Input: part model. Units: mm. Frame: model coordinates. Face numbers are marked on the shaded views. A direction names the side the tool comes from. Coordinates: 2 decimals unless noted, no trailing zeros. Write each loop counter-clockwise with the first axis right and the second up, starting at its lowest first coordinate (ties: lowest second). Pieces come first, ordered by that corner, then holes. Notation, with made-up numbers: (12, -1) - (70, -1) arc R16 cw to (70, 29) - close; hole circle Ø8 at (34.25, -13.75). An arc over 180 degrees is marked (long way). One line per question, with ' | ' between items. Start each with the question number.
1) First-contact query: P1, Ø5.5, axis at x = 0, y = 12, coming from the -Z side; P2, Ø1.2, axis at x = -24, y = 24, coming from the -Z side. Flat tips, straight axial feed; report the tip coordinate or a pass-through.
2) Section query D-D on x = -26.5. Return loops of the section in (y, z).
3) Draft query along Y for the marked faces 1, 2 and 3. Return one class per face: released by +Y, released by -Y, zero draft, split by the parting line, or undercut.
4) Section query A-A on y = 24. Return loops of the section in (x, z) (3 decimals), and give its area (3 significant figures).
5) Section query C-C on z = 4. Give the number of separate pieces and of enclosed holes in the cut face, and give its area (3 significant figures).
6) Reachability of the marked faces 4 and 5 from +Z, -Z, +X, -X, +Y, -Y: full face, straight path, thin tool, end or side. Return the list, or none.
7) Line query: line 1 (Y direction, x = -24, z = 4.75) (3 decimals); line 2 (Y direction, x = -24, z = 0.8); line 3 (X direction, y = 3, z = 1.5). Output: solid intervals per line, ascending.
8) Section query B-B on x = -12. Return loops of the section in (y, z) (3 decimals), and give its area (3 significant figures).
```python
from build123d import *

# Parameters (mm, degrees)
SKETCH1_W           = 40
SKETCH1_H           = 40
SKETCH1_R           = 4.55
BOSS_EXTRUDE1_DEPTH = 1.6
SKETCH2_W           = 40
SKETCH2_H           = 40
SKETCH2_R           = 1.025
BOSS_EXTRUDE2_DEPTH = 15


with BuildPart() as part:
    # Sketch1 → Boss-Extrude1 (new body)
    with BuildSketch(Plane(origin=(0, 0, 0), x_dir=(0, 1, 0), z_dir=(0, 0, 1))):
        with Locations((12, 12)):
            Rectangle(SKETCH1_W, SKETCH1_H)
        with Locations(Location((0, 0, 0), (0, 0, 270))):
            Circle(SKETCH1_R, mode=Mode.SUBTRACT)
        with Locations(Location((12, 0, 0), (0, 0, 270))):
            Circle(SKETCH1_R, mode=Mode.SUBTRACT)
        with Locations(Location((24, 0, 0), (0, 0, 270))):
            Circle(SKETCH1_R, mode=Mode.SUBTRACT)
        with Locations(Location((12, 12, 0), (0, 0, 270))):
            Circle(SKETCH1_R, mode=Mode.SUBTRACT)
        with Locations(Location((24, 12, 0), (0, 0, 270))):
            Circle(SKETCH1_R, mode=Mode.SUBTRACT)
        with Locations(Location((12, 24, 0), (0, 0, 270))):
            Circle(SKETCH1_R, mode=Mode.SUBTRACT)
        with Locations(Location((24, 24, 0), (0, 0, 270))):
            Circle(SKETCH1_R, mode=Mode.SUBTRACT)
        with Locations(Location((0, 12, 0), (0, 0, 270))):
            Circle(SKETCH1_R, mode=Mode.SUBTRACT)
        with Locations(Location((0, 24, 0), (0, 0, 270))):
            Circle(SKETCH1_R, mode=Mode.SUBTRACT)
    extrude(amount=BOSS_EXTRUDE1_DEPTH)

    # Sketch2 → Boss-Extrude2 (add)
    with BuildSketch(Plane.XY.offset(1.6)):
        with Locations((-12, 12)):
            Rectangle(SKETCH2_W, SKETCH2_H)
        Circle(SKETCH2_R, mode=Mode.SUBTRACT)
        with Locations((-12, 0)):
            Circle(SKETCH2_R, mode=Mode.SUBTRACT)
        with Locations((-24, 0)):
            Circle(SKETCH2_R, mode=Mode.SUBTRACT)
        with Locations((-12, 12)):
            Circle(SKETCH2_R, mode=Mode.SUBTRACT)
        with Locations((-24, 12)):
            Circle(SKETCH2_R, mode=Mode.SUBTRACT)
        with Locations((-12, 24)):
            Circle(SKETCH2_R, mode=Mode.SUBTRACT)
        with Locations((-24, 24)):
            Circle(SKETCH2_R, mode=Mode.SUBTRACT)
        with Locations((0, 12)):
            Circle(SKETCH2_R, mode=Mode.SUBTRACT)
        with Locations((0, 24)):
            Circle(SKETCH2_R, mode=Mode.SUBTRACT)
    extrude(amount=BOSS_EXTRUDE2_DEPTH)


solid = part.part
```
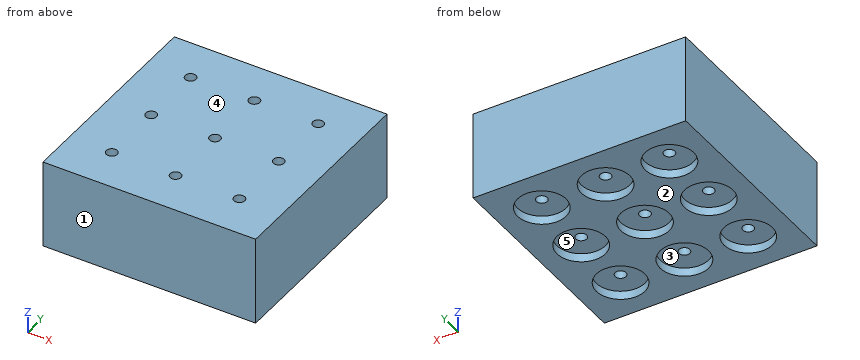
Answer key:
1) P1: z = 1.6 | P2: through
2) outline: (-8, 0) - (-3.8, 0) - (-3.8, 1.6) - (3.8, 1.6) - (3.8, 0) - (8.2, 0) - (8.2, 1.6) - (15.8, 1.6) - (15.8, 0) - (20.2, 0) - (20.2, 1.6) - (27.8, 1.6) - (27.8, 0) - (32, 0) - (32, 16.6) - (-8, 16.6) - close
3) face 1: released by -Y | face 2: zero draft | face 3: undercut
4) outline: (-32, 0) - (-28.55, 0) - (-28.55, 1.6) - (-25.025, 1.6) - (-25.025, 16.6) - (-32, 16.6) - close; (-22.975, 1.6) - (-19.45, 1.6) - (-19.45, 0) - (-16.55, 0) - (-16.55, 1.6) - (-13.025, 1.6) - (-13.025, 16.6) - (-22.975, 16.6) - close; (-10.975, 1.6) - (-7.45, 1.6) - (-7.45, 0) - (-4.55, 0) - (-4.55, 1.6) - (-1.025, 1.6) - (-1.025, 16.6) - (-10.975, 16.6) - close; (1.025, 1.6) - (4.55, 1.6) - (4.55, 0) - (8, 0) - (8, 16.6) - (1.025, 16.6) - close | area: 528 mm²
5) separate pieces: 1 | enclosed holes: 9 | area: 1,570 mm²
6) face 4: +Z, +X, -X, +Y, -Y | face 5: -Z
7) line 1: -8 to -1.025, 1.025 to 10.975, 13.025 to 22.975, 25.025 to 32 | line 2: -8 to -4.55, 4.55 to 7.45, 16.55 to 19.45, 28.55 to 32 | line 3: -32 to -27.42, -20.58 to -15.42, -8.58 to -3.42, 3.42 to 8
8) outline: (-8, 0) - (-4.55, 0) - (-4.55, 1.6) - (-1.025, 1.6) - (-1.025, 16.6) - (-8, 16.6) - close; (1.025, 1.6) - (4.55, 1.6) - (4.55, 0) - (7.45, 0) - (7.45, 1.6) - (10.975, 1.6) - (10.975, 16.6) - (1.025, 16.6) - close; (13.025, 1.6) - (16.55, 1.6) - (16.55, 0) - (19.45, 0) - (19.45, 1.6) - (22.975, 1.6) - (22.975, 16.6) - (13.025, 16.6) - close; (25.025, 1.6) - (28.55, 1.6) - (28.55, 0) - (32, 0) - (32, 16.6) - (25.025, 16.6) - close | area: 528 mm²
